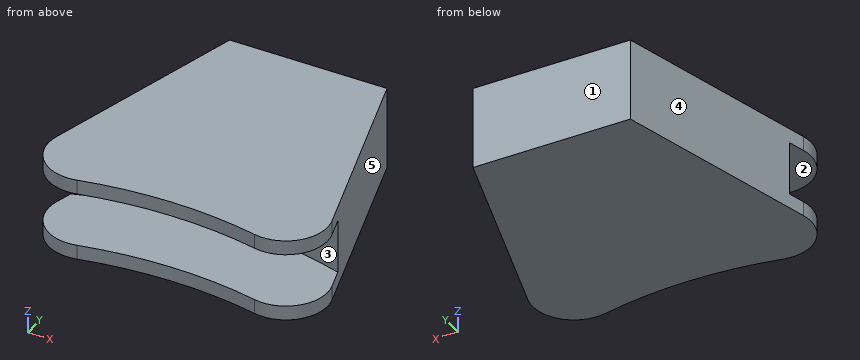
from build123d import *

# Parameters (mm, degrees)
BOSS_EXTRUDE1_DEPTH = 10
SKETCH5_W           = 13
SKETCH5_H           = 100
FILLET1_R           = 10


with BuildPart() as part:
    # Sketch1 → Boss-Extrude1 (new body, symmetric)
    with BuildSketch(Plane.XY):
        with BuildLine():
            Line((17.04861701, 0), (36.638934873, -67.52052444))
            ThreePointArc((36.638934873, -67.52052444), (-1.647556066, -60.00028765), (-39.897531443, -67.704100565))
            Line((-39.897531443, -67.704100565), (-20.95138299, 0))
            Line((-20.95138299, 0), (17.04861701, 0))
        make_face()
    extrude(amount=BOSS_EXTRUDE1_DEPTH, both=True)

    # Sketch5 → Cut-Revolve2 (revolve, cut)
    with BuildSketch(Plane(origin=(0, 0, 0), x_dir=(0, 0, -1), z_dir=(1, 0, 0))):
        with Locations((0, -190)):
            Rectangle(SKETCH5_W, SKETCH5_H)
    revolve(axis=Axis((0, -140, 0), (0, 0, -1)), mode=Mode.SUBTRACT)

    # Fillet1
    fillet1_edges = [part.edges().sort_by_distance(p)[0] for p in [
        (36.638934873, -67.52052444, -8.25),
        (-39.897531443, -67.704100565, -8.25),
        (-39.897531443, -67.704100565, 8.25),
        (36.638934873, -67.52052444, 8.25),
    ]]
    fillet(fillet1_edges, radius=FILLET1_R)


solid = part.part
The listing builds one solid part. Answer for the finished solid, in the listing's coordinates (mm). Face numbers are marked on the shaded views. A direction names the side the tool comes from. Give positions to 0.01 mm unless a question says otherwise; leave off trailing zeros. Loops run counter-clockwise (first coordinate to the right, second up) from the corner with the lowest first, then second, coordinate; pieces in that order, holes last. Notation, with made-up numbers: M 21.25,79 L 55.25,79 A23 ccw 55.25,87 Z; hole C 50.25,-39 d9. An arc over 180 degrees is marked long. Answer as CSV lines item,"result".
Item 1: The part is cut by section A-A (x = -16.5). Give the vertices of the cut face in (y, z).
Values follow:
outline,"M -61.15,-10 L 0,-10 L 0,10 L -61.15,10 L -61.15,6.5 L -41.37,6.5 L -41.37,-6.5 L -61.15,-6.5 Z"
Item 2: The part is cut by section D-D (x = 9). Give the vertices of the cut face in (y, z).
Values follow:
outline,"M -60.54,-10 L 0,-10 L 0,10 L -60.54,10 L -60.54,6.5 L -40.41,6.5 L -40.41,-6.5 L -60.54,-6.5 Z"
Item 3: Given pin 1 Ø10 at (y, z) = (-11, 6.5) entering from +X; pin 2 Ø10 at (y, z) = (-19.5, 4) entering from -X, each flat-ended and moving along its own axis, determine where each tip first touches the part or whether it passes through.
Values follow:
pin 1,"stops at x = 21.69"
pin 2,"stops at x = -27.81"
Item 4: Which of the six approach directions +Z, -Z, +X, -X, +Y, -Y give full straight-line access (tool end or side, diameter ignored) to the marked faces 1 and 2?
Values follow:
face 1,"+Z, -Z, +X, -X, +Y"
face 2,"-Y"
Item 5: The part is cut by section C-C (y = -8). Give the vertices of the cut face in (x, z), and give its area (3 significant figures).
Values follow:
outline,"M -23.19,-10 L 19.37,-10 L 19.37,10 L -23.19,10 Z"
area,"851 mm^2"
Item 6: Straight lines are drawn through the part: line 1 along Z through (x, y) = (-2, -51.5); line 2 along X through (y, z) = (-16, 3.75); line 3 along X through (y, z) = (-24.5, 4.75). For each, find the intervals that lie inside material, in ascending order. Write a range as [from, to].
Values follow:
line 1,"z = [-10, -6.5], [6.5, 10]"
line 2,"x = [-25.43, 21.69]"
line 3,"x = [-27.81, 24.16]"
Item 7: The part is cut by section B-B (z = 3.75). Give the vertices of the cut face in (x, y), and give its area (3 significant figures).
Values follow:
outline,"M -33.79,-45.88 A100 cw 29.99,-44.6 L 17.05,0 L -20.95,0 Z"
area,"2,080 mm^2"
Item 8: The mould has two halves that part along X. Classify the marked faces 3, 4 and 5: released by +X, released by -X, zero draft, split by the parting line, or undercut.
Values follow:
face 3,"undercut"
face 4,"released by -X"
face 5,"released by +X"
